Work out the finished part from the listing and answer in its coordinate system (mm). A direction names the side the tool comes from. Round coordinates to 2 decimals unless told otherwise and drop trailing zeros. Order: outer loops, then holes, each group sorted by start corner. A loop starts at its lowest first (then second) coordinate and runs counter-clockwise, first axis right, second up. Notation, with made-up numbers: (-15, 73.5) - (18, 73.5) arc R21 cw to (18, 78.5) - close; hole circle Ø3 at (18.5, 22). An arc over 180 degrees is marked (long way). Use one line per item in the form item = value. Start each with the question number.
Q1. For a pull along Y with two mould halves and no side action, classify faces 1 (the cylindrical face through (60.93, 1.45, 1.83)), 2 (the flat face through (-41.732, 4, 36)), 3 (the flat face through (-45, 74.422, 4)), 4 (the flat face through (58, 8.33, 36)) as +Y half, -Y half, draft (parallel to the pull), parting line (faces both ways), or undercut.
Q2. The part is cut by section C-C on y = 25.5. Determine the outline of the cut face in (x, z), plus the area to 3 significant figures.
Q3. Which of the six approach directions +Z, -Z, +X, -X, +Y, -Y give full straight-line access (tool end or side, diameter ignored) to faces 5 (the flat face through (58, 67.022, 36)), 6 (the cylindrical face through (-49.126, 39.266, 59.71)), 7 (the flat face through (7, 7.366, -13)), 8 (the flat face through (5, 37, -53.964)), 9 (the flat face through (7, 37, 53.964))?
Q4. The part is cut by section D-D on z = -13. Determine the outline of the cut face in (x, y).
Q5. The part is cut by section B-B on z = 29. Determine the outline of the cut face in (x, y).
Q6. The part is cut by section A-A on x = 39.5. Determine the outline of the cut face in (y, z).
Q7. Find the intervals of material crossed by line 1 (Z direction, x = 52, y = 65); line 2 (X direction, y = 58.5, z = 9.5); line 3 (Z direction, x = 41.5, y = 6), in increasing order. Write a range as [from, to].
from build123d import *

# Parameters (mm, degrees)
F0_W     = 113.10765706
F0_H     = 115.1223033667
F1_DEPTH = 74.422
F2_W     = 95.2637083828
F2_H     = 35.6879141182
F3_DEPTH = 127.762
F4_W     = 58.8790695183
F4_H     = 35.6879141182
F5_DEPTH = 78.486
F6_W     = 58.6911616847
F6_H     = 35.1123027503
F7_DEPTH = 72.898
F8_W     = 95.1198078692
F8_H     = 64.1806852072
F9_DEPTH = 67.056
F10_R    = 5.08
F11_R    = 5.08


with BuildPart() as f1:
    # F0 (on Front) → F1 (new body)
    with BuildSketch(Plane.XZ):
        with Locations((5.9000151232, 3.5975724459)):
            Rectangle(F0_W, F0_H)
    extrude(amount=-F1_DEPTH)

    # F2 (on Front) → F3 (cut)
    with BuildSketch(Plane.XZ):
        with Locations((5.9000197798, 36.1196221784)):
            Rectangle(F2_W, F2_H)
    extrude(amount=-F3_DEPTH, mode=Mode.SUBTRACT)

    # F4 (on Right) → F5 (cut)
    with BuildSketch(Plane.YZ):
        with Locations((36.9658360723, 36.1196221784)):
            Rectangle(F4_W, F4_H)
    extrude(amount=-F5_DEPTH, mode=Mode.SUBTRACT)

    # F6 (on face) → F7 (cut)
    with BuildSketch(Plane.YZ.offset(62.4538436532)):
        with Locations((37.6759679057, 36.4074278623)):
            Rectangle(F6_W, F6_H)
    extrude(amount=-F7_DEPTH, mode=Mode.SUBTRACT)

    # F8 (on face) → F9 (cut)
    with BuildSketch(Plane(origin=(0, 74.422, 0), x_dir=(-1, 0, 0), z_dir=(0, 1, 0))):
        with Locations((-5.9719700366, -13.8146774843)):
            Rectangle(F8_W, F8_H)
    extrude(amount=-F9_DEPTH, mode=Mode.SUBTRACT)

    # F10
    f10_edges = [f1.edges().sort_by_distance(p)[0] for p in [
        (-50.653813, 0, 3.597572),
    ]]
    fillet(f10_edges, radius=F10_R)

    # F11
    f11_edges = [f1.edges().sort_by_distance(p)[0] for p in [
        (62.453844, 0, 3.597572),
        (8.440015, 0, 61.158724),
        (62.453844, 37.211, 61.158724),
    ]]
    fillet(f11_edges, radius=F11_R)


solid = f1.part
Found:
q1.face_1 = -Y half
q1.face_2 = draft
q1.face_3 = +Y half
q1.face_4 = undercut
q2.outline = (-50.65, -53.96) - (62.45, -53.96) - (62.45, 18.85) - (53.53, 18.85) - (53.53, -45.91) - (-41.59, -45.91) - (-41.59, 18.28) - (-50.65, 18.28) - close; (-50.65, 53.96) - (62.45, 53.96) - (62.45, 56.08) arc R5.08 ccw to (57.37, 61.16) - (-45.57, 61.16) arc R5.08 ccw to (-50.65, 56.08) - close
q2.area = 2,870 mm²
q3.face_5 = +X
q3.face_6 = +Z, -X, +Y, -Y
q3.face_7 = +Y
q3.face_8 = -Z, +X, -X, +Y, -Y
q3.face_9 = none
q4.outline = (-50.65, 5.08) arc R5.08 ccw to (-45.57, 0) - (57.37, 0) arc R5.08 ccw to (62.45, 5.08) - (62.45, 74.42) - (53.53, 74.42) - (53.53, 7.37) - (-41.59, 7.37) - (-41.59, 74.42) - (-50.65, 74.42) - close
q5.outline = (-50.65, 5.08) arc R5.08 ccw to (-45.57, 0) - (-41.73, 0) - (-41.73, 7.53) - (-50.65, 7.53) - close; (-50.65, 66.41) - (-41.73, 66.41) - (-41.73, 74.42) - (-50.65, 74.42) - close; (53.53, 0) - (57.37, 0) arc R5.08 ccw to (62.45, 5.08) - (62.45, 8.33) - (53.53, 8.33) - close; (53.53, 67.02) - (62.45, 67.02) - (62.45, 74.42) - (53.53, 74.42) - close
q6.outline = (0, -53.96) - (74.42, -53.96) - (74.42, -45.91) - (7.37, -45.91) - (7.37, 18.28) - (0, 18.28) - close; (0, 53.96) - (74.42, 53.96) - (74.42, 61.16) - (5.08, 61.16) arc R5.08 ccw to (0, 56.08) - close
q7.line_1 = [-53.96, -45.91], [53.96, 61.16]
q7.line_2 = [-50.65, -41.59], [53.53, 62.45]
q7.line_3 = [-53.96, 18.28], [53.96, 61.16]
